from build123d import *

# Parameters (mm, degrees)
MODEL_R             = 2.1
MODEL_R_2           = 3.4
BOSS_EXTRUDE1_DEPTH = 400


with BuildPart() as part:
    # Model → Boss-Extrude1 (new body)
    with BuildSketch(Plane.XY):
        with BuildLine():
            Line((13, -11), (15, -11))
            Line((15, -11), (15, 11))
            Line((15, 11), (13, 11))
            Line((13, 11), (13, 6.75))
            Line((13, 6.75), (9.664213562, 6.75))
            Line((9.664213562, 6.75), (6, 10.414213562))
            Line((6, 10.414213562), (6, 14.480384758))
            Line((6, 14.480384758), (5.7, 15))
            Line((5.7, 15), (6, 15.519615242))
            Line((6, 15.519615242), (6, 19.585786438))
            Line((6, 19.585786438), (9.664213562, 23.25))
            Line((9.664213562, 23.25), (13, 23.25))
            Line((13, 23.25), (13, 19))
            Line((13, 19), (15, 19))
            Line((15, 19), (15, 28))
            ThreePointArc((15, 28), (14.414213562, 29.414213562), (13, 30))
            Line((13, 30), (4, 30))
            Line((4, 30), (4, 28))
            Line((4, 28), (8.25, 28))
            Line((8.25, 28), (8.25, 24.664213562))
            Line((8.25, 24.664213562), (4.585786438, 21))
            Line((4.585786438, 21), (0.519615242, 21))
            Line((0.519615242, 21), (0, 20.7))
            Line((0, 20.7), (-0.519615242, 21))
            Line((-0.519615242, 21), (-4.585786438, 21))
            Line((-4.585786438, 21), (-8.25, 24.664213562))
            Line((-8.25, 24.664213562), (-8.25, 28))
            Line((-8.25, 28), (-4, 28))
            Line((-4, 28), (-4, 30))
            Line((-4, 30), (-13, 30))
            ThreePointArc((-13, 30), (-14.414213562, 29.414213562), (-15, 28))
            Line((-15, 28), (-15, 19))
            Line((-15, 19), (-13, 19))
            Line((-13, 19), (-13, 23.25))
            Line((-13, 23.25), (-9.664213562, 23.25))
            Line((-9.664213562, 23.25), (-6, 19.585786438))
            Line((-6, 19.585786438), (-6, 15.519615242))
            Line((-6, 15.519615242), (-5.7, 15))
            Line((-5.7, 15), (-6, 14.480384758))
            Line((-6, 14.480384758), (-6, 10.414213562))
            Line((-6, 10.414213562), (-9.664213562, 6.75))
            Line((-9.664213562, 6.75), (-13, 6.75))
            Line((-13, 6.75), (-13, 11))
            Line((-13, 11), (-15, 11))
            Line((-15, 11), (-15, -11))
            Line((-15, -11), (-13, -11))
            Line((-13, -11), (-13, -6.75))
            Line((-13, -6.75), (-9.664213562, -6.75))
            Line((-9.664213562, -6.75), (-6, -10.414213562))
            Line((-6, -10.414213562), (-6, -14.480384758))
            Line((-6, -14.480384758), (-5.7, -15))
            Line((-5.7, -15), (-6, -15.519615242))
            Line((-6, -15.519615242), (-6, -19.585786438))
            Line((-6, -19.585786438), (-9.664213562, -23.25))
            Line((-9.664213562, -23.25), (-13, -23.25))
            Line((-13, -23.25), (-13, -19))
            Line((-13, -19), (-15, -19))
            Line((-15, -19), (-15, -28))
            ThreePointArc((-15, -28), (-14.414213562, -29.414213562), (-13, -30))
            Line((-13, -30), (-4, -30))
            Line((-4, -30), (-4, -28))
            Line((-4, -28), (-8.25, -28))
            Line((-8.25, -28), (-8.25, -24.664213562))
            Line((-8.25, -24.664213562), (-4.585786438, -21))
            Line((-4.585786438, -21), (-0.519615242, -21))
            Line((-0.519615242, -21), (0, -20.7))
            Line((0, -20.7), (0.519615242, -21))
            Line((0.519615242, -21), (4.585786438, -21))
            Line((4.585786438, -21), (8.25, -24.664213562))
            Line((8.25, -24.664213562), (8.25, -28))
            Line((8.25, -28), (4, -28))
            Line((4, -28), (4, -30))
            Line((4, -30), (13, -30))
            ThreePointArc((13, -30), (14.414213562, -29.414213562), (15, -28))
            Line((15, -28), (15, -19))
            Line((15, -19), (13, -19))
            Line((13, -19), (13, -23.25))
            Line((13, -23.25), (9.664213562, -23.25))
            Line((9.664213562, -23.25), (6, -19.585786438))
            Line((6, -19.585786438), (6, -15.519615242))
            Line((6, -15.519615242), (5.7, -15))
            Line((5.7, -15), (6, -14.480384758))
            Line((6, -14.480384758), (6, -10.414213562))
            Line((6, -10.414213562), (9.664213562, -6.75))
            Line((9.664213562, -6.75), (13, -6.75))
            Line((13, -6.75), (13, -11))
        make_face()
        with Locations((11.6, -26.6)):
            Circle(MODEL_R, mode=Mode.SUBTRACT)
        with Locations((11.6, 26.6)):
            Circle(MODEL_R, mode=Mode.SUBTRACT)
        with Locations((0, 15)):
            Circle(MODEL_R_2, mode=Mode.SUBTRACT)
        with Locations((0, -15)):
            Circle(MODEL_R_2, mode=Mode.SUBTRACT)
        with Locations((-11.6, 26.6)):
            Circle(MODEL_R, mode=Mode.SUBTRACT)
        with Locations((-11.6, -26.6)):
            Circle(MODEL_R, mode=Mode.SUBTRACT)
        with BuildLine():
            Line((-8.835786438, 4.75), (-12, 4.75))
            ThreePointArc((-12, 4.75), (-12.707106781, 4.457106781), (-13, 3.75))
            Line((-13, 3.75), (-13, -3.75))
            ThreePointArc((-13, -3.75), (-12.707106781, -4.457106781), (-12, -4.75))
            Line((-12, -4.75), (-8.835786438, -4.75))
            Line((-8.835786438, -4.75), (-3.651792162, -9.933994275))
            ThreePointArc((-3.651792162, -9.933994275), (-3.470780421, -10.020243754), (-3.275866822, -9.973202156))
            ThreePointArc((-3.275866822, -9.973202156), (-2e-08, -9), (3.275866789, -9.973202134))
            ThreePointArc((3.275866789, -9.973202134), (3.470780401, -10.020243756), (3.651792162, -9.933994275))
            Line((3.651792162, -9.933994275), (8.835786438, -4.75))
            Line((8.835786438, -4.75), (12, -4.75))
            ThreePointArc((12, -4.75), (12.707106781, -4.457106781), (13, -3.75))
            Line((13, -3.75), (13, 3.75))
            ThreePointArc((13, 3.75), (12.707106781, 4.457106781), (12, 4.75))
            Line((12, 4.75), (8.835786438, 4.75))
            Line((8.835786438, 4.75), (3.651792162, 9.933994275))
            ThreePointArc((3.651792162, 9.933994275), (3.470780421, 10.020243754), (3.275866822, 9.973202156))
            ThreePointArc((3.275866822, 9.973202156), (2e-08, 9), (-3.275866789, 9.973202134))
            ThreePointArc((-3.275866789, 9.973202134), (-3.470780401, 10.020243756), (-3.651792162, 9.933994275))
            Line((-3.651792162, 9.933994275), (-8.835786438, 4.75))
        make_face(mode=Mode.SUBTRACT)
    extrude(amount=BOSS_EXTRUDE1_DEPTH)


solid = part.part
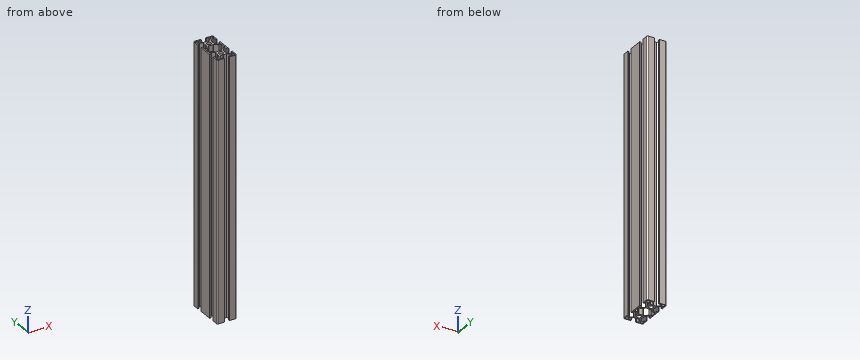
Here's how the part is built. I have some questions about the finished solid (model axes, mm). Coordinates: 2 decimals unless noted, no trailing zeros. Write each loop counter-clockwise with the first axis right and the second up, starting at its lowest first coordinate (ties: lowest second). Pieces come first, ordered by that corner, then holes.
Item 1: I want a section at A-A on y = 0.5. Write out the boundary of the cut face in (x, z).
Item 2: If I drill on line 1 (Y direction, x = 11.25, z = 148); line 2 (X direction, y = -10.5, z = 255); line 3 (X direction, y = 26.5, z = 263.5), over which ranges is the centre line in solid material (lowest first)?
Item 3: I want a section at B-B on z = 179.5. Count the separate pieces of the cut face and the enclosed holes in it, and give its area (3 significant figures).
Item 4: Will these pins go through, and if not, where does the flat tip stop? pin 1 (3.5 mm diameter, centred on y = 18, z = 264, fed in from -X); pin 2 (1 mm diameter, centred on x = 14, z = 112.5, fed in from +Y); pin 3 (1 mm diameter, centred on y = 15, z = 115.5, fed in from -X); pin 4 (1.2 mm diameter, centred on y = 12.5, z = 202.5, fed in from +X).
Findings below:
1. outline: (-15, 0) - (-13, 0) - (-13, 400) - (-15, 400) - close; (13, 0) - (15, 0) - (15, 400) - (13, 400) - close
2. line 1: y = -30 to -28.67, -24.53 to -23.25, -6.75 to -4.75, 4.75 to 6.75, 23.25 to 24.53, 28.67 to 30
2. line 2: x = -15 to -13, -6 to 6, 13 to 15
2. line 3: x = -15 to -13.7, -9.5 to -8.25, 8.25 to 9.5, 13.7 to 15
3. separate pieces: 1
3. enclosed holes: 7
3. area: 592 mm2
4. pin 1: stops at x = -15
4. pin 2: stops at y = 29.94
4. pin 3: stops at x = -5.99
4. pin 4: stops at x = 6
